Input: part model. Units: mm. Frame: model coordinates. A direction names the side the tool comes from. Coordinates: 2 decimals unless noted, no trailing zeros. Order: outer loops, then holes, each group sorted by start corner. A loop starts at its lowest first (then second) coordinate and runs counter-clockwise, first axis right, second up. Notation, with made-up numbers: M -4.75,47 L 21.25,47 A13 cw 21.25,68 Z; hole C 60.5,6.5 d5. An arc over 180 degrees is marked long. Answer in a Markdown table with one row per item.
from build123d import *

# Parameters (mm, degrees)
F1_DEPTH = 3.175


with BuildPart() as f1:
    # F0 (on Right) → F1 (new body)
    with BuildSketch(Plane.YZ):
        Polygon((-48.195562, 60.325), (-48.195562, 0), (-48.195562, -63.5), (-20.145495, -63.5), (-20.145495, -60.325), (7.904572, -60.325), (7.904572, -63.5), (43.879438, -63.5), (66.688176, -46.286863), (64.775605, -43.752558), (87.584343, -26.539421), (89.496914, -29.073725), (112.305652, -11.860588), (86.852017, 13.258684), (84.621845, 10.998826), (59.166806, 36.119484), (61.396978, 38.379342), (35.941938, 63.5), (7.904572, 63.5), (7.904572, 60.325), (-20.145495, 60.325), (-20.145495, 63.5), (-48.195562, 63.5), align=None)
    extrude(amount=F1_DEPTH)


solid = f1.part
1) Material intervals for probe 1 along Z at (x, y) = (2.15, 4.5) (3 decimals); probe 2 along Y at (x, z) = (0.2, -46); probe 3 along Z at (x, y) = (0.2, 43.5), sorted ascending.
Resolved:
| item | result |
|---|---|
| probe 1 | z = -60.325 to 60.325 |
| probe 2 | y = -48.2 to 66.47 |
| probe 3 | z = -63.5 to 56.04 |
2) Mould query, pull axis Y, two halves, no side actions, for faces 1 (the face through (2, -34, 63.5)), 2 (the face through (2, -6, -60.325)), 3 (the face through (2, -48.196, 1)), 4 (the face through (2, -20.145, -62)). Classes: +Y half, -Y half, draft (parallel to the pull), parting line (faces both ways), or undercut.
Resolved:
| item | result |
|---|---|
| face 1 | draft |
| face 2 | undercut |
| face 3 | -Y half |
| face 4 | undercut |
3) Contact query for flat-ended pins moving along their axis: pin 1 (1 mm diameter, centred on x = 2.5, z = -62.5, fed in from +Y); pin 2 (1.6 mm diameter, centred on x = 2, z = 62, fed in from +Y); pin 3 (1.5 mm diameter, centred on x = 2, y = 57, fed in from +Z). Output: stop coordinate, or through.
Resolved:
| item | result |
|---|---|
| pin 1 | stops at y = 45.87 |
| pin 2 | stops at y = 38.27 |
| pin 3 | stops at z = 43.46 |
4) Cut plane A-A, the plane x = 2.1. Output: boundary loops of the cut face in (y, z) (1 decimal), and give its area (3 significant figures).
Resolved:
| item | result |
|---|---|
| outline | M -48.2,-63.5 L -20.1,-63.5 L -20.1,-60.3 L 7.9,-60.3 L 7.9,-63.5 L 43.9,-63.5 L 66.7,-46.3 L 64.8,-43.8 L 87.6,-26.5 L 89.5,-29.1 L 112.3,-11.9 L 86.9,13.3 L 84.6,11 L 59.2,36.1 L 61.4,38.4 L 35.9,63.5 L 7.9,63.5 L 7.9,60.3 L -20.1,60.3 L -20.1,63.5 L -48.2,63.5 Z |
| area | 15,400 mm2 |
5) Cut plane C-C, the plane y = -2. Output: boundary loops of the cut face in (x, z) (3 decimals).
Resolved:
| item | result |
|---|---|
| outline | M 0,-60.325 L 3.175,-60.325 L 3.175,60.325 L 0,60.325 Z |
6) Reachability of faces 5 (the face through (2, 7.905, 62)), 6 (the face through (2, 7.905, -62)), 7 (the face through (1.57, 48.85, 50.76)) from +Z, -Z, +X, -X, +Y, -Y: full face, straight path, thin tool, end or side. Return the list, or none.
Resolved:
| item | result |
|---|---|
| face 5 | +Z, +X, -X |
| face 6 | -Z, +X, -X |
| face 7 | +Z, +X, -X, +Y |
7) Cut plane B-B, the plane z = 41. Output: boundary loops of the cut face in (x, y) (3 decimals), and give its area (3 significant figures).
Resolved:
| item | result |
|---|---|
| outline | M 0,-48.196 L 3.175,-48.196 L 3.175,58.741 L 0,58.741 Z |
| area | 340 mm2 |
